Can you work these out from the drawing? Everything is in mm from the part's minimum corner. A direction names the side the tool comes from. Give positions to 0.01 mm unless a question says otherwise; leave off trailing zeros. Order: outer loops, then holes, each group sorted by start corner. A loop starts at its lowest first (then second) coordinate and runs counter-clockwise, first axis right, second up. Notation, with made-up numbers: M 3,-21.5 L 49,-21.5 A25 cw 49,8.5 Z; hole C -4,-28 d5. An arc over 180 degrees is marked long. Use a Markdown table: item, result. Add a question column.
Item 1: Suppose I cut it at A-A on z = 1. Write out the boundary of the cut face in (x, y), plus the area to 3 significant figures.
Item 2: Suppose I cut it at C-C on y = 4. Write out the boundary of the cut face in (x, z).
Item 3: If I drill on L1, parallel to X at y = 3.5, z = 13.5; L2, parallel to Y at x = 15, z = 11.5; L3, parallel to Y at x = 15, z = 5.5, over which ranges is the centre line in solid material (lowest first)? Write a range as from..to.
Item 4: If we mould it in two halves opening along X, with no side actions, what happens to the marked faces 3, 4 and 5? For each: released by +X, released by -X, zero draft, split by the parting line, or undercut.
Item 5: Suppose I cut it at B-B on z = 4. Write out the boundary of the cut face in (x, y).
Item 6: For the marked faces 1 and 2, which set-ups out of +Z, -Z, +X, -X, +Y, -Y let a thin tool reach every point of the face, with its end or its side?
Item 7: Suppose I cut it at D-D on x = 12. Write out the boundary of the cut face in (y, z), plus the area to 3 significant figures.
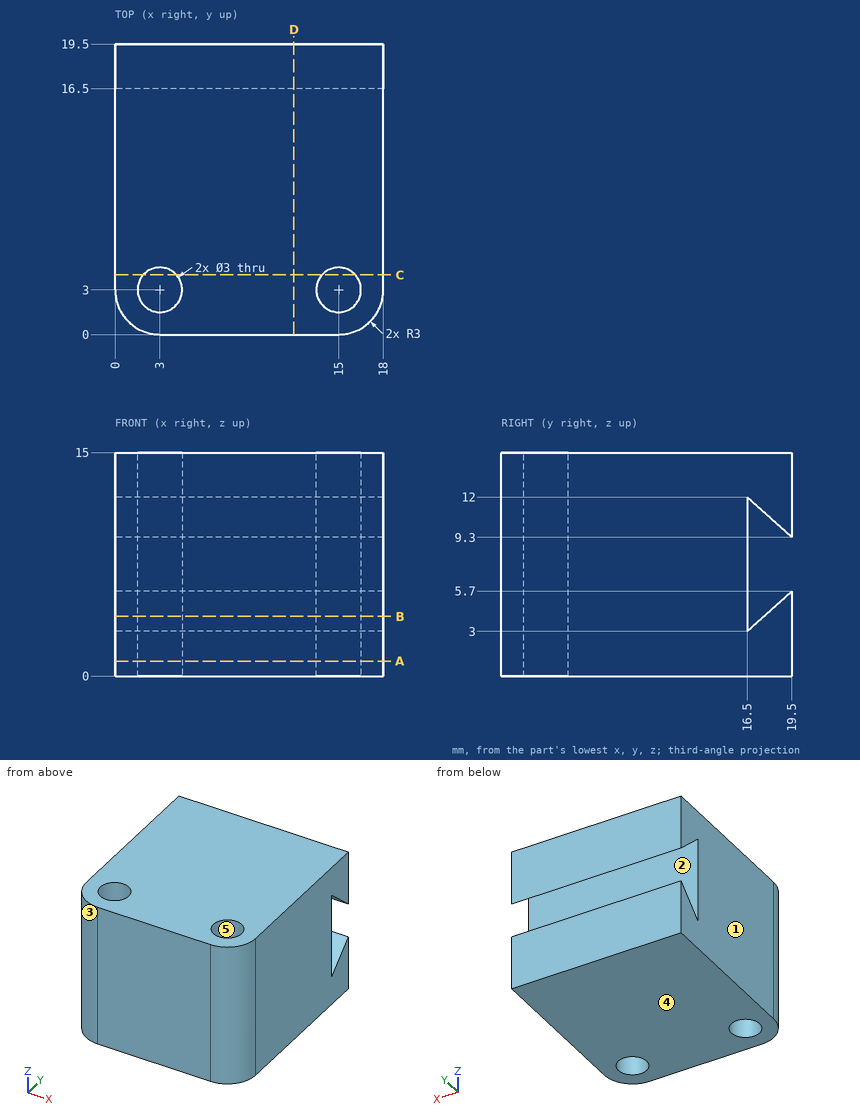
Findings below:
| question | item | result |
|---|---|---|
| 1 | outline | M 0,3 A3 ccw 3,0 L 15,0 A3 ccw 18,3 L 18,19.5 L 0,19.5 Z; hole C 3,3 d3; hole C 15,3 d3 |
| 1 | area | 333 mm^2 |
| 2 | outline | M 0,0 L 1.88,0 L 1.88,15 L 0,15 Z; M 4.12,0 L 13.88,0 L 13.88,15 L 4.12,15 Z; M 16.12,0 L 18,0 L 18,15 L 16.12,15 Z |
| 3 | L1 | x = 0..1.59, 4.41..13.59, 16.41..18 |
| 3 | L2 | y = 0..1.5, 4.5..16.5, 17.06..19.5 |
| 3 | L3 | y = 0..1.5, 4.5..16.5, 19.28..19.5 |
| 4 | face 3 | released by -X |
| 4 | face 4 | zero draft |
| 4 | face 5 | undercut |
| 5 | outline | M 0,3 A3 ccw 3,0 L 15,0 A3 ccw 18,3 L 18,16.5 L 0,16.5 Z; M 0,17.61 L 18,17.61 L 18,19.5 L 0,19.5 Z; hole C 3,3 d3; hole C 15,3 d3 |
| 6 | face 1 | +Z, -Z, -X, +Y, -Y |
| 6 | face 2 | +X, -X |
| 7 | outline | M 0,0 L 19.5,0 L 19.5,5.7 L 16.5,3 L 16.5,12 L 19.5,9.3 L 19.5,15 L 0,15 Z |
| 7 | area | 274 mm^2 |
